Solid Edge part; units mm, degrees
sketch "Sketch1" plane through (0, 0, 0) normal (0, -1, 0) x (1, 0, 0)
  line L0 (0, 0) -> (-89.6999, -93.0601)
  line L1 (-75.4219, -107.064) -> (31.4288, 0)
  line L2 (31.4288, 0) -> (0, 0)
  arc A0 (-75.4219, -107.064) -> (-89.6999, -93.0601) centre (-82.5, -100) cw
extrude "Protrusion1" add sketch "Sketch1" along normal blind 4
sketch "Sketch2" plane through (-30.5356, 0, -55) normal (0, 1, 0) x (-0.7064012, 0, -0.7078117)
  circle A0 centre (68.5592, 4.9929) radius 7.5
extrude "Cutout1" cut sketch "Sketch2" against normal up to next
sketch "Sketch3" plane through (-30.5356, -4, -55) normal (0, -1, 0) x (0.7064012, 0, 0.7078117)
  line L0 (58.3766, 15.1194) -> (56.3339, 17.1662)
  line L1 (56.3339, 17.1662) -> (60.5, 17.2386)
  line L2 (60.5, 17.2386) -> (58.3766, 15.1194)
extrude "Cutout2" cut sketch "Sketch3" against normal up to next
properties material "Stainless steel"
Can you work these out from the model? Positions are in its coordinate system, mm. Give positions to 0.01 mm unless a question says otherwise; leave off trailing zeros. Loops run counter-clockwise (first coordinate to the right, second up) from the corner with the lowest first, then second, coordinate; pieces in that order, holes last. Notation, with made-up numbers: M 3,29.5 L 22,29.5 A22 cw 22,50.5 Z; hole C 81,7.5 d1. An arc over 180 degrees is marked long. Use one line per item in the form item = value. Start each with the question number.
(1) I want a section at B-B, the plane y = -0.65. Write out the boundary of the cut face in (x, z), and give its area (3 significant figures).
(2) I'm going to push flat-ended pins straight in: P1, Ø1, axis at y = -2.5, z = -19, coming from the +X side; P2, Ø1, axis at y = -3, z = -71, coming from the -X side; P3, Ø1, axis at y = -2.5, z = -40.5, coming from the +X side; P4, Ø13.5, axis at x = -82.5, z = -100, coming from the +Y side. Where does each tip first touch, or does it pass through?
(3) I want a section at A-A, the plane z = -100. Write out the boundary of the cut face in (x, y), and give its area (3 significant figures).
(4) I want a section at D-D, the plane x = -20.5. Write out the boundary of the cut face in (y, z).
(5) Thinking about a two-plate mould opening in X: for faces 1 (the cylindrical face through (-87, -2, -94)), 2 (the flat face through (-22.744, -1.972, -54.281)), 3 (the flat face through (-30, 0, -51)), which applies, released by +X, released by -X, zero draft, split by the parting line, or undercut?
(6) Please list where these lines run through material, in increasing order: line 1 (X direction, y = -1.8, z = -18); line 2 (Z direction, x = -60, y = -1); line 3 (X direction, y = -3.25, z = -33.5).
(7) I want a section at C-C, the plane x = -82.5. Write out the boundary of the cut face in (y, z).
Worked out:
q1.outline = M -89.7,-93.06 A10 ccw -75.42,-107.06 L 31.43,0 L 0,0 L 0,-3 L -2.89,-3 Z; hole C -82.5,-100 d15
q1.area = 2,950 mm²
q2.P1 = 12.97
q2.P2 = -68.92
q2.P3 = -8.49
q2.P4 = through
q3.outline = M -92.5,-4 L -90,-4 L -90,0 L -92.5,0 Z; M -75,-4 L -68.37,-4 L -68.37,0 L -75,0 Z
q3.area = 36.5 mm²
q4.outline = M -4,-52.03 L 0,-52.03 L 0,-21.27 L -4,-21.27 Z
q5.face_1 = undercut
q5.face_2 = released by +X
q5.face_3 = zero draft
q6.line_1 = -17.35 to 13.46
q6.line_2 = -91.61 to -62.25
q6.line_3 = -32.29 to -2
q7.outline = M -4,-110 L 0,-110 L 0,-107.5 L -4,-107.5 Z; M -4,-92.5 L 0,-92.5 L 0,-85.59 L -4,-85.59 Z
